```python
from build123d import *

# Parameters (mm, degrees)
F0_W     = 60
F0_H     = 100
F1_DEPTH = 3
F3_D     = 8.8
F4_T     = -2.5


with BuildPart() as f1:
    # F0 (on Front) → F1 (new body)
    with BuildSketch(Plane.XZ):
        Rectangle(F0_W, F0_H)
    extrude(amount=F1_DEPTH)

    # F3 (through all)
    with Locations(Plane.XZ.offset(3)):
        with Locations((-9.7982781008, 25.4148039967), (14.2741240561, 27.5341067463), (14.0938721597, -23.4790239483), (-12.2754974291, -26.1800661683)):
            Hole(F3_D / 2)

    # F4
    f4_openings = [f1.faces().sort_by_distance(p)[0] for p in [
        (-0.0665, -3, -0.034758),
    ]]
    offset(amount=F4_T, openings=f4_openings)


solid = f1.part
```
The model under review builds one solid part; all positions refer to its coordinate system, in mm. A direction names the side the tool comes from. Round coordinates to 2 decimals unless told otherwise and drop trailing zeros. Order: outer loops, then holes, each group sorted by start corner. A loop starts at its lowest first (then second) coordinate and runs counter-clockwise, first axis right, second up. Notation, with made-up numbers: (58, 78) -> (78, 78) arc R23 cw to (78, 106) -> close; hole circle Ø8 at (0.25, 39). An arc over 180 degrees is marked (long way). Use a Markdown table: item, result.
Q1. Tool access review of faces 4 (the cylindrical face through (-18.65, -2.75, -28.82)), 5 (the flat face through (-30, -1, -1)): name each direction out of +Z, -Z, +X, -X, +Y, -Y from which nothing blocks a thin tool from reaching the whole face with its end or side.
Values:
| item | result |
|---|---|
| face 4 | -Y |
| face 5 | +Z, -Z, -X, +Y, -Y |
Q2. We need section A-A on z = -36. Write out the cut boundary in (x, y).
Values:
| item | result |
|---|---|
| outline | (-30, -3) -> (-27.5, -3) -> (-27.5, -2.5) -> (27.5, -2.5) -> (27.5, -3) -> (30, -3) -> (30, 0) -> (-30, 0) -> close |
Q3. We need section D-D on x = 12. Write out the cut boundary in (y, z).
Values:
| item | result |
|---|---|
| outline | (-3, -50) -> (0, -50) -> (0, -27.35) -> (-3, -27.35) -> (-3, -30.05) -> (-2.5, -30.05) -> (-2.5, -47.5) -> (-3, -47.5) -> close; (-3, -19.61) -> (0, -19.61) -> (0, 23.77) -> (-3, 23.77) -> (-3, 21.02) -> (-2.5, 21.02) -> (-2.5, -16.9) -> (-3, -16.9) -> close; (-3, 31.3) -> (0, 31.3) -> (0, 50) -> (-3, 50) -> (-3, 47.5) -> (-2.5, 47.5) -> (-2.5, 34.05) -> (-3, 34.05) -> close |
Q4. We need section B-B on y = -1.25. Write out the cut boundary in (x, z).
Values:
| item | result |
|---|---|
| outline | (-30, -50) -> (30, -50) -> (30, 50) -> (-30, 50) -> close; hole circle Ø8.8 at (-12.28, -26.18); hole circle Ø8.8 at (-9.8, 25.41); hole circle Ø8.8 at (14.09, -23.48); hole circle Ø8.8 at (14.27, 27.53) |
Q5. Clearance check with a flat-ended pin moving along its axis: P1, Ø8, axis at x = 13, z = 12, coming from the -Y side. State where the tip first meets the part, or that it passes through.
Values:
| item | result |
|---|---|
| P1 | stops at y = -2.5 |
Q6. We need section C-C on z = 28.5. Write out the cut boundary in (x, y), then the cut area to 3 significant figures.
Values:
| item | result |
|---|---|
| outline | (-30, -3) -> (-27.5, -3) -> (-27.5, -2.5) -> (-15.97, -2.5) -> (-15.97, -3) -> (-12.94, -3) -> (-12.94, 0) -> (-30, 0) -> close; (-6.66, -3) -> (-3.63, -3) -> (-3.63, -2.5) -> (7.44, -2.5) -> (7.44, -3) -> (9.98, -3) -> (9.98, 0) -> (-6.66, 0) -> close; (18.57, -3) -> (21.11, -3) -> (21.11, -2.5) -> (27.5, -2.5) -> (27.5, -3) -> (30, -3) -> (30, 0) -> (18.57, 0) -> close |
| area | 121 mm^2 |
Q7. Mouldability with a two-part tool opening along Z and no side actions: class faces 1 (the cylindrical face through (20.987, -2.746, -23.176)), 2 (the flat face through (0, -1, 50)), 3 (the flat face through (0, 0, 1)) as +Z half, -Z half, draft (parallel to the pull), parting line (faces both ways), or undercut.
Values:
| item | result |
|---|---|
| face 1 | undercut |
| face 2 | +Z half |
| face 3 | draft |
Q8. For line 1 (Z direction, x = 14, y = -1.15); line 2 (X direction, y = -2.55, z = 10); line 3 (Z direction, x = -10.5, y = -2.45), list the stretches that pass through material, from the lowest coordinate up.
Values:
| item | result |
|---|---|
| line 1 | z = -50 to -27.88, -19.08 to 23.14, 31.93 to 50 |
| line 2 | x = -30 to -27.5, 27.5 to 30 |
| line 3 | z = -50 to -30.21, -22.15 to 21.07, 29.76 to 50 |
